```python
from build123d import *

# Parameters (mm, degrees)
SKETCH_1_R               = 15
EXTRUDE_1_DEPTH          = 42
SKETCH_2_R               = 7
CUT_EXTRUDE_1_DEPTH      = 20
SKETCH_3_R               = 5
CUT_EXTRUDE_2_DEPTH      = 20
SKETCH_5_R               = 2
CUT_EXTRUDE_3_DEPTH      = 20
CUT_EXTRUDE_3_DEPTH_BACK = 10


with BuildPart() as part:
    # 草图1 → 凸台-拉伸1 (new body)
    with BuildSketch(Plane.XY):
        with Locations((0, -2.373543689)):
            Circle(SKETCH_1_R)
    extrude(amount=EXTRUDE_1_DEPTH)

    # 草图2 → 切除-拉伸1 (cut)
    with BuildSketch(Plane.XY.offset(42)):
        with Locations((0, -2.373543689)):
            Circle(SKETCH_2_R)
    extrude(amount=-CUT_EXTRUDE_1_DEPTH, mode=Mode.SUBTRACT)

    # 草图3 → 切除-拉伸2 (cut)
    with BuildSketch(Plane(origin=(0, 0, 0), x_dir=(-1, 0, 0), z_dir=(0, 0, -1))):
        with Locations((0, -2.373543689)):
            Circle(SKETCH_3_R)
    extrude(amount=-CUT_EXTRUDE_2_DEPTH, mode=Mode.SUBTRACT)

    # 草图5 → 切除-拉伸3 (cut, two sides)
    with BuildSketch(Plane(origin=(0, 10, 0), x_dir=(1, 0, 0), z_dir=(0, 1, 0))) as cut_extrude_3_sk:
        with Locations((0, -5.037121645)):
            Circle(SKETCH_5_R)
    extrude(amount=CUT_EXTRUDE_3_DEPTH, mode=Mode.SUBTRACT)
    extrude(cut_extrude_3_sk.sketch, amount=-CUT_EXTRUDE_3_DEPTH_BACK, mode=Mode.SUBTRACT)


solid = part.part
```
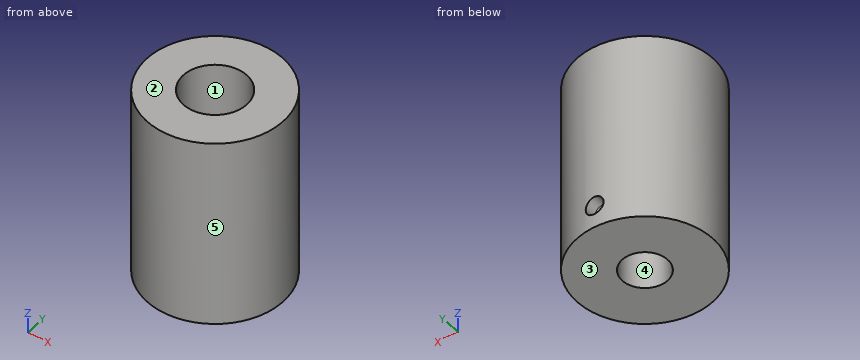
Geometry check sheet. Reference: the model listing, model coordinates, mm. Face numbers are marked on the shaded views. A direction names the side the tool comes from. Give positions to 0.01 mm unless a question says otherwise; leave off trailing zeros. Write each loop counter-clockwise with the first axis right and the second up, starting at its lowest first coordinate (ties: lowest second). Pieces come first, ordered by that corner, then holes.
1) Material ranges on L1, parallel to Z at x = 0, y = 6; L2, parallel to Y at x = 0, z = 13.5; L3, parallel to Y at x = 0, z = 34, recorded low to high.
2) Section check A-A, the plane x = 0. Record the boundary of the cut face in (y, z), and give its area (3 significant figures).
3) Section check C-C, the plane y = 5.5. Record the boundary of the cut face in (x, z), and give its area (3 significant figures).
4) Access from +Z, -Z, +X, -X, +Y, -Y to the whole of each face (thin tool, end or side, straight path). Record for the marked faces 1 and 2.
5) Section check D-D, the plane z = 13.5. Record the boundary of the cut face in (x, y).
6) Gauge pin test, flat ends, axial feed: pin 1 (7 mm diameter, centred on x = 0, y = -4.5, fed in from +Z); pin 2 (3 mm diameter, centred on y = -12, z = 29.5, fed in from -X); pin 3 (12 mm diameter, centred on y = -14, z = 16, fed in from -X). Record the tip position at first contact, or that the pin passes through.
7) Release check for a two-part mould opening along X. For the marked faces 3, 4 and 5 record: pulls with the +X half, pulls with the -X half, needs draft (parallel to the pull), parting line crosses it, or undercut.
8) Section check B-B, the plane y = -6.5. Record the boundary of the cut face in (x, z).
Computed:
1. L1: z = 0 to 3.04, 7.04 to 42
1. L2: y = -17.37 to -7.37, 2.63 to 12.63
1. L3: y = -17.37 to -9.37, 4.63 to 12.63
2. outline: (-17.37, 0) - (-7.37, 0) - (-7.37, 20) - (2.63, 20) - (2.63, 7.04) - (12.63, 7.04) - (12.63, 42) - (4.63, 42) - (4.63, 22) - (-9.37, 22) - (-9.37, 42) - (-17.37, 42) - close; (2.63, 0) - (12.63, 0) - (12.63, 3.04) - (2.63, 3.04) - close
2. area: 740 mm2
3. outline: (-12.77, 0) - (12.77, 0) - (12.77, 42) - (-12.77, 42) - close; hole circle Ø4 at (0, 5.04)
3. area: 1,060 mm2
4. face 1: +Z
4. face 2: +Z, +X, -X, +Y, -Y
5. outline: circle Ø30 at (0, -2.37); hole circle Ø10 at (0, -2.37)
6. pin 1: stops at z = 22
6. pin 2: stops at x = -12.61
6. pin 3: stops at x = -13.9
7. face 3: needs draft
7. face 4: undercut
7. face 5: parting line crosses it
8. outline: (-14.42, 0) - (-2.82, 0) - (-2.82, 20) - (2.82, 20) - (2.82, 0) - (14.42, 0) - (14.42, 42) - (5.65, 42) - (5.65, 22) - (-5.65, 22) - (-5.65, 42) - (-14.42, 42) - close
